Could you check a few things on this model? Use its own coordinates, in mm. A direction names the side the tool comes from. Coordinates: 2 decimals unless noted, no trailing zeros. Order: outer loops, then holes, each group sorted by start corner. A loop starts at its lowest first (then second) coordinate and runs counter-clockwise, first axis right, second up. Notation, with made-up numbers: (55, -36) - (82, -36) arc R18 cw to (82, -16) - close; hole circle Ø5 at (58, 27.5). An arc over 180 degrees is marked (long way). One line per item, written item: value.
from build123d import *

# Parameters (mm, degrees)
BOSS_EXTRUDE1_DEPTH = 2.5
BOSS_EXTRUDE2_DEPTH = 3.75
SKETCH3_R           = 2.5
BOSS_EXTRUDE3_DEPTH = 2.5


with BuildPart() as part:
    # Sketch1 → Boss-Extrude1 (new, symmetric)
    with BuildSketch(Plane.XY):
        Polygon((-17.5, 25), (-5, 37.5), (-5, 30.428932188), (-12.5, 22.928932188), (-12.5, 5), (-17.5, 5), align=None)
    boss_extrude1 = extrude(amount=BOSS_EXTRUDE1_DEPTH, both=True)

    # Sketch1_3 → Boss-Extrude2 (add, symmetric)
    with BuildSketch(Plane.XY):
        Polygon((-20, 5), (-20, 0), (0, 0), (0, 5), (-12.5, 5), (-17.5, 5), align=None)
    boss_extrude2 = extrude(amount=BOSS_EXTRUDE2_DEPTH, both=True)

    # Sketch3 → Boss-Extrude3 (add)
    with BuildSketch(Plane.XZ):
        with Locations(Location((-15, 0, 0), (0, 0, 90))):
            Circle(SKETCH3_R)
    boss_extrude3 = extrude(amount=BOSS_EXTRUDE3_DEPTH)

    # Mirror1: Boss-Extrude1, Boss-Extrude2, Boss-Extrude3 across plane
    add(boss_extrude1.mirror(Plane(origin=(0, 0, 0), x_dir=(0, 0, 1), z_dir=(1, 0, 0))))
    add(boss_extrude2.mirror(Plane(origin=(0, 0, 0), x_dir=(0, 0, 1), z_dir=(1, 0, 0))))
    add(boss_extrude3.mirror(Plane(origin=(0, 0, 0), x_dir=(0, 0, 1), z_dir=(1, 0, 0))))


solid = part.part
Item 1: I want a section at D-D on z = 0. Please give me the cut outline in (x, y), then the cut area to 3 significant figures.
Conclusion:
outline: (-20, 0) - (-17.5, 0) - (-17.5, -2.5) - (-12.5, -2.5) - (-12.5, 0) - (12.5, 0) - (12.5, -2.5) - (17.5, -2.5) - (17.5, 0) - (20, 0) - (20, 5) - (17.5, 5) - (17.5, 25) - (5, 37.5) - (5, 30.43) - (12.5, 22.93) - (12.5, 5) - (-12.5, 5) - (-12.5, 22.93) - (-5, 30.43) - (-5, 37.5) - (-17.5, 25) - (-17.5, 5) - (-20, 5) - close
area: 556 mm²
Item 2: I want a section at A-A on y = 22. Please give me the cut outline in (x, z), then the cut area to 3 significant figures.
Conclusion:
outline: (-17.5, -2.5) - (-12.5, -2.5) - (-12.5, 2.5) - (-17.5, 2.5) - close; (12.5, -2.5) - (17.5, -2.5) - (17.5, 2.5) - (12.5, 2.5) - close
area: 50.0 mm²
Item 3: I want a section at B-B on x = -6. Please give me the cut outline in (y, z), then the cut area to 3 significant figures.
Conclusion:
outline: (0, -3.75) - (5, -3.75) - (5, 3.75) - (0, 3.75) - close; (29.43, -2.5) - (36.5, -2.5) - (36.5, 2.5) - (29.43, 2.5) - close
area: 72.9 mm²
Item 4: For faces 4 (the face through (13, 21, 2.5)), 5 (the face through (-17.5, 15, 0)), 6 (the face through (12.5, 14, 0)), 7 (the face through (17.5, 15, 0)), which set-ups out of +Z, -Z, +X, -X, +Y, -Y let a thin tool reach every point of the face, with its end or its side?
Conclusion:
face 4: +Z, +X, -X, +Y
face 5: +Z, -Z, -X, +Y
face 6: +Z, -Z
face 7: +Z, -Z, +X, +Y
Item 5: If I drill on probe 1 along X at (y, z) = (14.5, -2); probe 2 along Z at (x, y) = (16, 10); probe 3 along Y at (x, z) = (-16.5, -3), over which ranges is the centre line in solid material (lowest first)?
Conclusion:
probe 1: -17.5 to -12.5, 12.5 to 17.5
probe 2: -2.5 to 2.5
probe 3: 0 to 5
Item 6: Thinking about a two-plate mould opening in Y: for faces 1 (the face through (-12.5, 14, 0)), 2 (the face through (13, 21, -2.5)), 3 (the face through (-11.3, 31.2, 0)), which applies, pulls with the +Y half, pulls with the -Y half, needs draft (parallel to the pull), parting line crosses it, or undercut?
Conclusion:
face 1: undercut
face 2: needs draft
face 3: pulls with the +Y half
Item 7: I want a section at C-C on x = -13. Please give me the cut outline in (y, z).
Conclusion:
outline: (-2.5, -1.5) - (0, -1.5) - (0, -3.75) - (5, -3.75) - (5, -2.5) - (29.5, -2.5) - (29.5, 2.5) - (5, 2.5) - (5, 3.75) - (0, 3.75) - (0, 1.5) - (-2.5, 1.5) - close
Item 8: I'm going to push flat-ended pins straight in: pin 1 Ø2 at (x, z) = (9.5, -1.5) entering from +Y; pin 2 Ø1.5 at (y, z) = (33, -0.5) entering from +X; pin 3 Ø1.5 at (y, z) = (13.5, -1) entering from +X; pin 4 Ø2 at (x, y) = (-0.5, 5.5) entering from -Z. Where does each tip first touch, or does it pass through?
Conclusion:
pin 1: y = 34
pin 2: x = 10.25
pin 3: x = 17.5
pin 4: z = -3.75
